Here's how the part is built. I have some questions about the finished solid (model axes, mm). Face numbers are marked on the shaded views. Coordinates: 2 decimals unless noted, no trailing zeros. Order: outer loops, then holes, each group sorted by start corner. A loop starts at its lowest first (then second) coordinate and runs counter-clockwise, first axis right, second up. Notation, with made-up numbers: M 29,-10 L 45,-10 A19 cw 45,4 Z; hole C 56.5,-19 d1. An arc over 180 degrees is marked long. One line per question, with ' | ' between items. Start each with the question number.
```python
from build123d import *

# Parameters (mm, degrees)
F0_W     = 63.5
F0_H     = 50.8
F0_R     = 4.1656
F0_R_2   = 14.2875
F1_DEPTH = 6.35


with BuildPart() as f1:
    # F0 (on Top) → F1 (new body)
    with BuildSketch(Plane.XY):
        Rectangle(F0_W, F0_H)
        with Locations((-26.1874, 0)):
            Circle(F0_R, mode=Mode.SUBTRACT)
        Circle(F0_R_2, mode=Mode.SUBTRACT)
        with Locations((26.1874, 0)):
            Circle(F0_R, mode=Mode.SUBTRACT)
    extrude(amount=-F1_DEPTH)


solid = f1.part
```
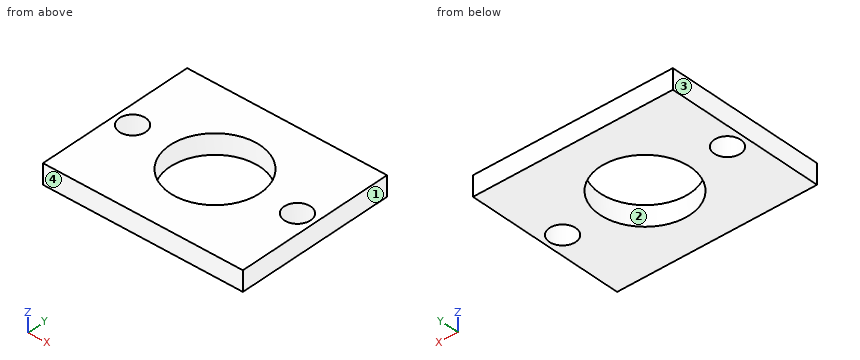
1. I need wall thicknesses on line 1 (Y direction, x = -26, z = -5); line 2 (X direction, y = -3, z = -5.5); line 3 (Y direction, x = 2, z = -2). Which ranges of each line are inside material? Lowest first, please.
2. Imagine slicing it at A-A (z = -5). Count the separate pieces of the cut face and the enclosed holes in it, then the cut area to 3 significant figures.
3. Imagine slicing it at B-B (x = 0). List the corners of the cut face in (y, z) for me.
4. Imagine slicing it at C-C (y = 0). List the corners of the cut face in (x, z) for me.
5. We'd pull the mould along X, two halves only. Please class the marked faces 1, 2, 3 and 4: released by +X, released by -X, zero draft, split by the parting line, or undercut.
6. Will this pin go through, and if not, where does the flat tip stop? pin 1 (6.5 mm diameter, centred on x = 26.19, y = 0, fed in from -Z).
7. Imagine slicing it at D-D (x = -7.5). List the corners of the cut face in (y, z) for me, then the cut area to 3 significant figures.
Entries:
1) line 1: -25.4 to -4.16, 4.16 to 25.4 | line 2: -31.75 to -29.08, -23.3 to -13.97, 13.97 to 23.3, 29.08 to 31.75 | line 3: -25.4 to -14.15, 14.15 to 25.4
2) separate pieces: 1 | enclosed holes: 3 | area: 2,480 mm²
3) outline: M -25.4,-6.35 L -14.29,-6.35 L -14.29,0 L -25.4,0 Z; M 14.29,-6.35 L 25.4,-6.35 L 25.4,0 L 14.29,0 Z
4) outline: M -31.75,-6.35 L -30.35,-6.35 L -30.35,0 L -31.75,0 Z; M -22.02,-6.35 L -14.29,-6.35 L -14.29,0 L -22.02,0 Z; M 14.29,-6.35 L 22.02,-6.35 L 22.02,0 L 14.29,0 Z; M 30.35,-6.35 L 31.75,-6.35 L 31.75,0 L 30.35,0 Z
5) face 1: released by +X | face 2: undercut | face 3: released by -X | face 4: zero draft
6) pin 1: through
7) outline: M -25.4,-6.35 L -12.16,-6.35 L -12.16,0 L -25.4,0 Z; M 12.16,-6.35 L 25.4,-6.35 L 25.4,0 L 12.16,0 Z | area: 168 mm²
